Design review of the part built by this model. Coordinates are the model's own, in mm. Coordinates: 2 decimals unless noted, no trailing zeros. Write each loop counter-clockwise with the first axis right and the second up, starting at its lowest first coordinate (ties: lowest second). Pieces come first, ordered by that corner, then holes. Notation, with made-up numbers: M 24.5,-30 L 40.5,-30 A25 cw 40.5,-2 Z; hole C 83,-26.5 d4. An arc over 180 degrees is marked long. One line per question, with ' | ' between items.
from build123d import *

# Parameters (mm, degrees)
SKETCH008_W                     = 25
SKETCH008_H                     = 25
SKETCH008_R                     = 2
PAD007_DEPTH                    = 0.5
SKETCH009_W                     = 5
SKETCH009_H                     = 5
PAD008_DEPTH                    = 2.6
SKETCH009_LINEARPATTERN008_2_W  = 5
SKETCH009_LINEARPATTERN008_2_H  = 5
PAD008_LINEARPATTERN008_2_DEPTH = 2.6
SKETCH009_LINEARPATTERN008_3_W  = 5
SKETCH009_LINEARPATTERN008_3_H  = 5
PAD008_LINEARPATTERN008_3_DEPTH = 2.6
SKETCH009_LINEARPATTERN008_4_W  = 5
SKETCH009_LINEARPATTERN008_4_H  = 5
PAD008_LINEARPATTERN008_4_DEPTH = 2.6
LINEARPATTERN007_COUNT          = 4
LINEARPATTERN007_PITCH          = 7.8


with BuildPart() as part:
    # Sketch008 → Pad007 (new body)
    with BuildSketch(Plane.XY.offset(0.5)):
        Rectangle(SKETCH008_W, SKETCH008_H)
        with Locations((-7.9, 7.9)):
            Circle(SKETCH008_R, mode=Mode.SUBTRACT)
        with Locations((7.9, 7.9)):
            Circle(SKETCH008_R, mode=Mode.SUBTRACT)
        with Locations((7.9, -7.9)):
            Circle(SKETCH008_R, mode=Mode.SUBTRACT)
        with Locations((-7.9, -7.9)):
            Circle(SKETCH008_R, mode=Mode.SUBTRACT)
    extrude(amount=PAD007_DEPTH)

    # Sketch009 → Pad008 (join)
    with BuildSketch(Plane.XY.offset(3.2)):
        with Locations((-11.7, -11.7)):
            Rectangle(SKETCH009_W, SKETCH009_H)
    pad008 = extrude(amount=-PAD008_DEPTH)

    # Sketch009 LinearPattern008 2 → Pad008 LinearPattern008 2 (add)
    with BuildSketch(Plane(origin=(7.8, 0, 3.2), x_dir=(1, 0, 0), z_dir=(0, 0, 1))):
        with Locations((-11.7, -11.7)):
            Rectangle(SKETCH009_LINEARPATTERN008_2_W, SKETCH009_LINEARPATTERN008_2_H)
    pad008_linearpattern008_2 = extrude(amount=-PAD008_LINEARPATTERN008_2_DEPTH)

    # Sketch009 LinearPattern008 3 → Pad008 LinearPattern008 3 (add)
    with BuildSketch(Plane(origin=(15.6, 0, 3.2), x_dir=(1, 0, 0), z_dir=(0, 0, 1))):
        with Locations((-11.7, -11.7)):
            Rectangle(SKETCH009_LINEARPATTERN008_3_W, SKETCH009_LINEARPATTERN008_3_H)
    pad008_linearpattern008_3 = extrude(amount=-PAD008_LINEARPATTERN008_3_DEPTH)

    # Sketch009 LinearPattern008 4 → Pad008 LinearPattern008 4 (add)
    with BuildSketch(Plane(origin=(23.4, 0, 3.2), x_dir=(1, 0, 0), z_dir=(0, 0, 1))):
        with Locations((-11.7, -11.7)):
            Rectangle(SKETCH009_LINEARPATTERN008_4_W, SKETCH009_LINEARPATTERN008_4_H)
    pad008_linearpattern008_4 = extrude(amount=-PAD008_LINEARPATTERN008_4_DEPTH)

    # LinearPattern007: Pad008, Pad008 LinearPattern008 2, Pad008 LinearPattern008 3, Pad008 LinearPattern008 4 ×4
    with Locations(*[(0, i * LINEARPATTERN007_PITCH, 0) for i in range(1, LINEARPATTERN007_COUNT)]):
        add(pad008)
        add(pad008_linearpattern008_2)
        add(pad008_linearpattern008_3)
        add(pad008_linearpattern008_4)


solid = part.part
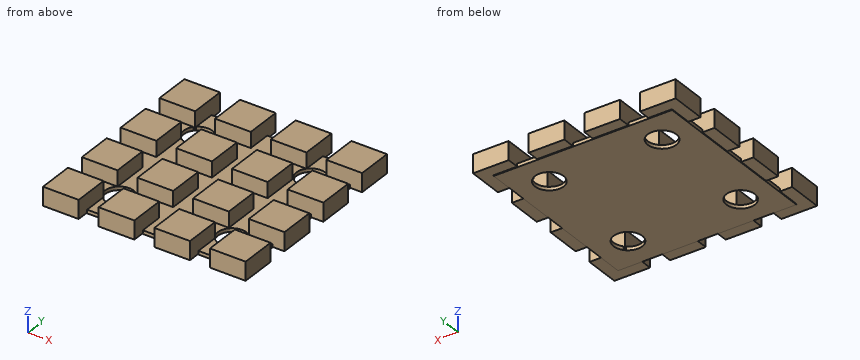
1. Take a section at D-D (z = 2.2). Count the separate pieces of the cut face and the enclosed holes in it, then the cut area to 3 significant figures.
Answer sheet:
separate pieces: 16 | enclosed holes: 0 | area: 400 mm^2
2. Take a section at A-A (x = 7.9). Write out the cut boundary in (y, z).
Answer sheet:
outline: M -12.5,0.5 L -9.9,0.5 L -9.9,1 L -12.5,1 Z; M -5.9,0.5 L 5.9,0.5 L 5.9,1 L -5.9,1 Z; M 9.9,0.5 L 12.5,0.5 L 12.5,1 L 9.9,1 Z
3. Take a section at C-C (y = 12). Write out the cut boundary in (x, z).
Answer sheet:
outline: M -14.2,0.6 L -12.5,0.6 L -12.5,0.5 L 12.5,0.5 L 12.5,0.6 L 14.2,0.6 L 14.2,3.2 L 9.2,3.2 L 9.2,1 L 6.4,1 L 6.4,3.2 L 1.4,3.2 L 1.4,1 L -1.4,1 L -1.4,3.2 L -6.4,3.2 L -6.4,1 L -9.2,1 L -9.2,3.2 L -14.2,3.2 Z
4. To check wall thickness, follow line 1 along Y through (x, z) = (9.5, 1.45); line 2 along Y through (x, z) = (7.9, 0.65). State the ranges of each line that lie inside material, in increasing order. Write a range as [from, to].
Answer sheet:
line 1: [-14.2, -9.2], [-6.4, -1.4], [1.4, 6.4], [9.2, 14.2] | line 2: [-12.5, -9.9], [-5.9, 5.9], [9.9, 12.5]
5. Insertion check: pin 1 Ø0.5 at (x, y) = (4.5, 13) entering from -Z; pin 2 Ø4 at (x, y) = (-0.5, -7) entering from +Z; pin 3 Ø0.8 at (x, y) = (-7, -11) entering from +Z. Each pin has a flat end and moves straight along its axis. Give the tip position at first contact, or say it passes through.
Answer sheet:
pin 1: z = 0.6 | pin 2: z = 3.2 | pin 3: z = 1
